Could you check a few things on this drawing? It's one solid part, dimensions in mm from its lowest x, y, z. Give positions to 0.01 mm unless a question says otherwise; leave off trailing zeros. Loops run counter-clockwise (first coordinate to the right, second up) from the corner with the lowest first, then second, coordinate; pieces in that order, holes last. Notation, with made-up numbers: M 73,-29.5 L 102,-29.5 A14 ccw 102,-5.5 Z; hole C 27.25,72 d10. An arc over 180 degrees is marked long. Return JSON: item names as keys, results as strings. Group by question number.
1. If we section it at A-A (x = 86.5): Write out the boundary of the cut face in (y, z).
2. If we section it at B-B (z = 37): Write out the boundary of the cut face in (x, y).
3. Please list where these lines run through material, in increasing order: line 1 (X direction, y = 0.8, z = 11); line 2 (Z direction, x = 117.5, y = 1.35).
4. For pin 1 (10 mm diameter, centred on x = 102.5, z = 55.5, fed in from +Y), with a flat end and sliding along its axis, tell me the tip position at first contact or that it passes through.
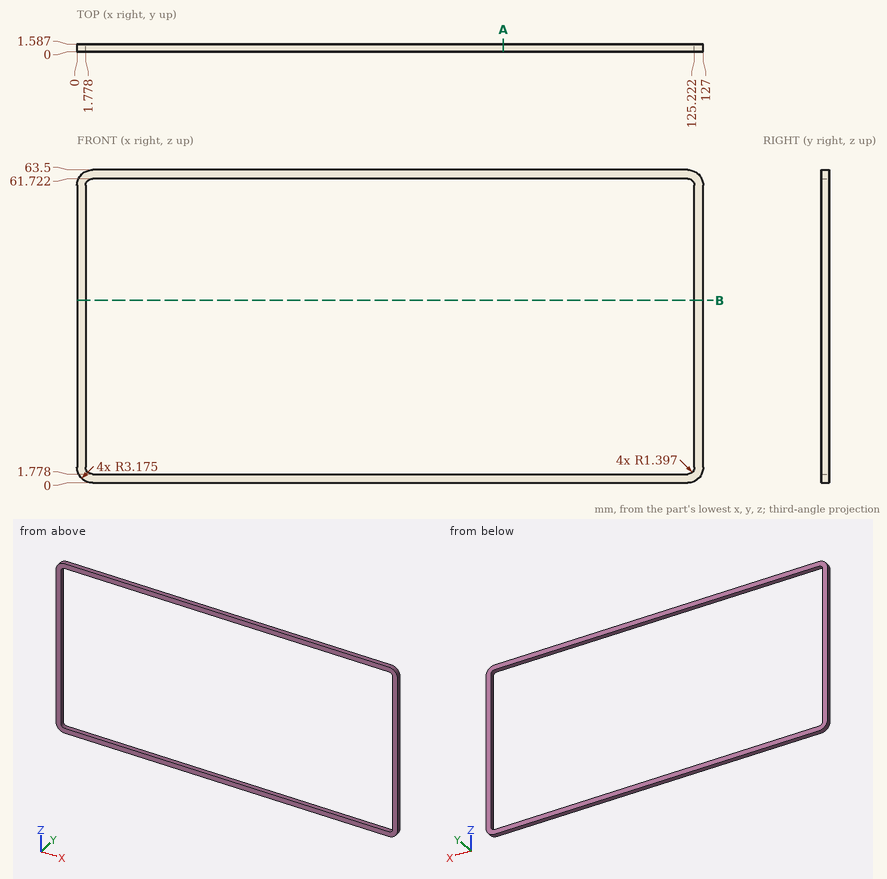
Answer:
{
 "1": {"outline": "M 0,0 L 1.59,0 L 1.59,1.78 L 0,1.78 Z; M 0,61.72 L 1.59,61.72 L 1.59,63.5 L 0,63.5 Z"},
 "2": {"outline": "M 0,0 L 1.78,0 L 1.78,1.59 L 0,1.59 Z; M 125.22,0 L 127,0 L 127,1.59 L 125.22,1.59 Z"},
 "3": {"line 1": "x = 0 to 1.78, 125.22 to 127", "line 2": "z = 0 to 1.78, 61.72 to 63.5"},
 "4": {"pin 1": "passes through"}
}
